Input: part model. Units: mm. Frame: model coordinates. A direction names the side the tool comes from. Give positions to 0.01 mm unless a question says otherwise; leave off trailing zeros. Order: outer loops, then holes, each group sorted by start corner. A loop starts at its lowest first (then second) coordinate and runs counter-clockwise, first axis right, second up. Notation, with made-up numbers: M -40,19 L -23,19 A6 cw -23,30 Z; hole C 78,-27.5 d5. An arc over 180 degrees is marked long. Use a Markdown table: item, result.
from build123d import *

# Parameters (mm, degrees)
F1_DEPTH  = 914.4
F10_W     = 1214.12
F10_H     = 604.52
F11_DEPTH = 12.7
F12_W     = 1214.12
F12_H     = 604.52
F13_DEPTH = 12.7


with BuildPart() as f1:
    # F0 (on Top) → F1 (new body)
    with BuildSketch(Plane.XY):
        Polygon((0, 38.1), (-3.175, 38.1), (-3.175, -3.175), (38.1, -3.175), (38.1, 0), (0, 0), align=None)
    extrude(amount=F1_DEPTH)


with BuildPart() as f4_1:
    # F4: instance of F1
    add(f1.part.mirror(Plane.YZ.offset(609.6)))


with BuildPart() as f5_1:
    # F5: instance of F4_1
    add(f4_1.part.mirror(Plane.XZ.offset(-304.8)))


with BuildPart() as f5_2:
    # F5: instance of F1
    add(f1.part.mirror(Plane.XZ.offset(-304.8)))


with BuildPart() as f1_1:
    add(f1.part)

    add(f4_1.part)  # F9 merges F4_1

    add(f5_1.part)  # F9 merges F5_1

    add(f5_2.part)  # F9 merges F5_2
    # F9: sweep along a path in F7
    with BuildLine(Plane.XY.offset(889)) as f9_path:
        Line((1219.2, 0), (0, 0))
        Line((0, 0), (0, 609.6))
        Line((0, 609.6), (1219.2, 609.6))
        Line((1219.2, 609.6), (1219.2, 0))
    # F8 (on face) → F9 (sweep)
    with BuildSketch(Plane.YZ.offset(38.1)):
        Polygon((2.54, 863.6), (0, 863.6), (0, 831.85), (2.54, 831.85), (2.54, 844.55), (7.62, 850.9), (2.54, 850.9), align=None)
        Polygon((2.54, 406.4), (0, 406.4), (0, 374.65), (2.54, 374.65), (2.54, 387.35), (7.62, 393.7), (2.54, 393.7), align=None)
    sweep(path=f9_path.line, transition=Transition.RIGHT)

    # F10 (on face) → F11 (join)
    with BuildSketch(Plane.XY.offset(850.9)):
        with Locations((609.6, 304.8)):
            Rectangle(F10_W, F10_H)
    extrude(amount=F11_DEPTH)

    # F12 (on face) → F13 (join)
    with BuildSketch(Plane.XY.offset(393.7)):
        with Locations((609.6, 304.8)):
            Rectangle(F12_W, F12_H)
    extrude(amount=F13_DEPTH)


solid = f1_1.part
1) Cut plane C-C on x = 889. Return loops of the section in (y, z).
Response values:
| item | result |
|---|---|
| outline | M 0,374.65 L 2.54,374.65 L 2.54,387.35 L 7.62,393.7 L 601.98,393.7 L 607.06,387.35 L 607.06,374.65 L 609.6,374.65 L 609.6,406.4 L 0,406.4 Z; M 0,831.85 L 2.54,831.85 L 2.54,844.55 L 7.62,850.9 L 601.98,850.9 L 607.06,844.55 L 607.06,831.85 L 609.6,831.85 L 609.6,863.6 L 0,863.6 Z |
2) Cut plane B-B on y = 121.5. Return loops of the section in (x, z), and give its area (3 significant figures).
Response values:
| item | result |
|---|---|
| outline | M 0,374.65 L 2.54,374.65 L 2.54,387.35 L 7.62,393.7 L 1211.58,393.7 L 1216.66,387.35 L 1216.66,374.65 L 1219.2,374.65 L 1219.2,406.4 L 0,406.4 Z; M 0,831.85 L 2.54,831.85 L 2.54,844.55 L 7.62,850.9 L 1211.58,850.9 L 1216.66,844.55 L 1216.66,831.85 L 1219.2,831.85 L 1219.2,863.6 L 0,863.6 Z |
| area | 31,200 mm² |
3) First-contact query: pin 1 Ø10 at (x, z) = (834, 838) entering from -Y; pin 2 Ø4 at (x, y) = (1053.5, 448) entering from +Z; pin 3 Ø12 at (x, y) = (968, 360) entering from -Z. Flat tips, straight axial feed; report the tip coordinate or a pass-through.
Response values:
| item | result |
|---|---|
| pin 1 | stops at y = 0 |
| pin 2 | stops at z = 863.6 |
| pin 3 | stops at z = 393.7 |
4) Cut plane A-A on z = 109. Return loops of the section in (x, y) (3 decimals), and give its area (3 significant figures).
Response values:
| item | result |
|---|---|
| outline | M -3.175,-3.175 L 38.1,-3.175 L 38.1,0 L 0,0 L 0,38.1 L -3.175,38.1 Z; M -3.175,571.5 L 0,571.5 L 0,609.6 L 38.1,609.6 L 38.1,612.775 L -3.175,612.775 Z; M 1181.1,-3.175 L 1222.375,-3.175 L 1222.375,38.1 L 1219.2,38.1 L 1219.2,0 L 1181.1,0 Z; M 1181.1,609.6 L 1219.2,609.6 L 1219.2,571.5 L 1222.375,571.5 L 1222.375,612.775 L 1181.1,612.775 Z |
| area | 1,010 mm² |
5) Material intervals for line 1 (Z direction, x = 1075.5, y = 289); line 2 (X direction, y = 28.5, z = 872) (3 decimals); line 3 (X direction, y = 51.5, z = 846), sorted ascending. Write a range as from..to.
Response values:
| item | result |
|---|---|
| line 1 | z = 393.7..406.4, 850.9..863.6 |
| line 2 | x = -3.175..0, 1219.2..1222.375 |
| line 3 | x = 0..3.7, 1215.5..1219.2 |
6) Reachability of faces 1 (the face through (618, 609.6, 848)), 2 (the face through (19, 0, 185)), 3 (the face through (1219.2, 19, 889)), 4 (the face through (0, 19, 616)) from +Z, -Z, +X, -X, +Y, -Y: full face, straight path, thin tool, end or side. Return the list, or none.
Response values:
| item | result |
|---|---|
| face 1 | +Z, -Z, +Y |
| face 2 | -Z |
| face 3 | +Z |
| face 4 | none |
7) Mould query, pull axis Z, two halves, no side actions, for faces 5 (the face through (-1, 601, 914.4)), 6 (the face through (1200, 609.6, 185)), 7 (the face through (1219.2, 591, 616)), 8 (the face through (-1, 601, 0)). Classes: released by +Z, released by -Z, zero draft, split by the parting line, or undercut.
Response values:
| item | result |
|---|---|
| face 5 | released by +Z |
| face 6 | zero draft |
| face 7 | undercut |
| face 8 | released by -Z |
